Geometry: see drawing. Coordinates: mm, zero at the bounding-box minimum. A direction names the side the tool comes from. Coordinates: 2 decimals unless noted, no trailing zeros. Order: outer loops, then holes, each group sorted by start corner. A loop starts at its lowest first (then second) coordinate and runs counter-clockwise, first axis right, second up. Notation, with made-up numbers: (43.5, 49) -> (100.5, 49) arc R16 cw to (100.5, 70) -> close; hole circle Ø4 at (84, 40.5). An arc over 180 degrees is marked (long way). Use one line per item in the form item = value.
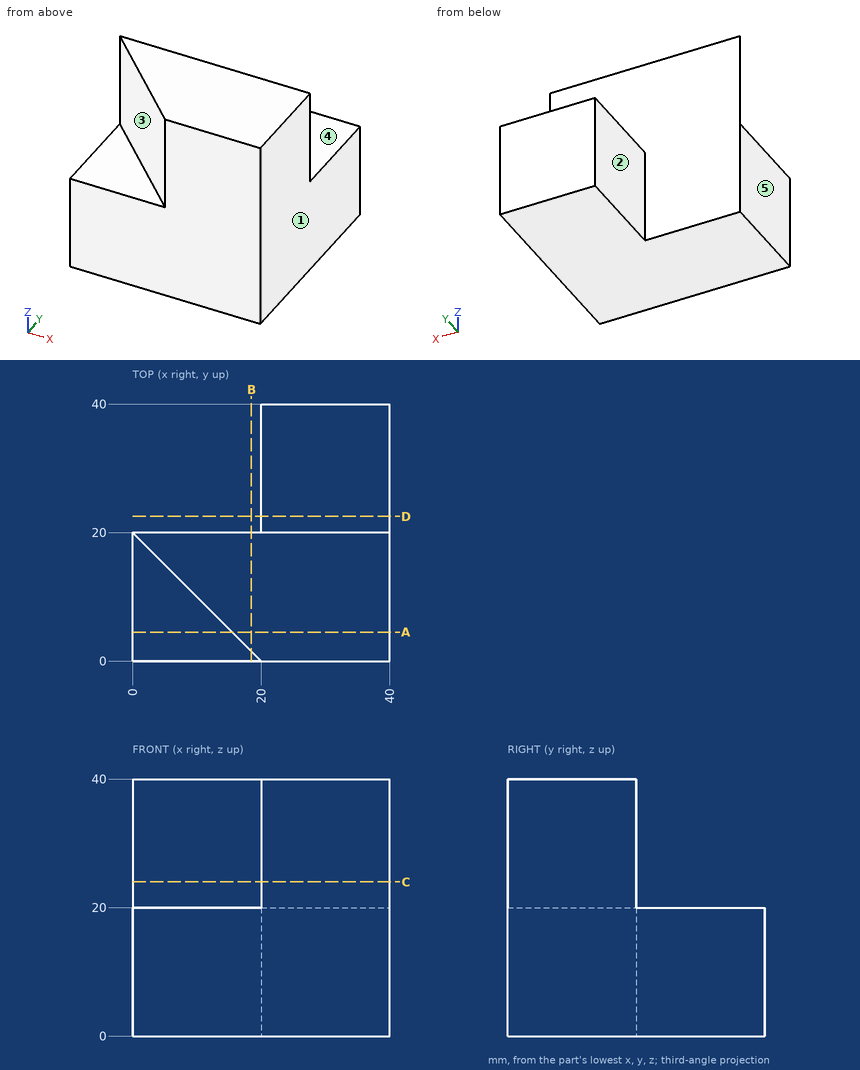
1) Contact query for flat-ended pins moving along their axis: P1, Ø16, axis at y = 31, z = 10.5, coming from the -X side; P2, Ø12, axis at x = 9.5, y = 6.5, coming from the -Z side; P3, Ø6, axis at x = 34, y = 25, coming from the +Z side; P4, Ø12, axis at y = 29.5, z = 30, coming from the -X side. Output: stop coordinate, or through.
Results found:
P1 = 20
P2 = 0
P3 = 20
P4 = through
2) Material intervals for probe 1 along Z at (x, y) = (11, 7.5); probe 2 along X at (y, z) = (27, 8.5), sorted ascending. Write a range as from..to.
Results found:
probe_1 = 0..20
probe_2 = 20..40
3) Section B-B, the plane x = 18.5. Output: boundary loops of the cut face in (y, z).
Results found:
outline = (0, 0) -> (20, 0) -> (20, 40) -> (1.5, 40) -> (1.5, 20) -> (0, 20) -> close
4) Access query for the marked faces 1, 2, 3, 4 and 5. Directions: +Z, -Z, +X, -X, +Y, -Y. A direction counts if a zero-diameter tool reaches every point of the face in a straight line with its end or side. Return the directions, or none.
Results found:
face_1 = +Z, -Z, +X, +Y, -Y
face_2 = +Z, -Z, -X, +Y
face_3 = +Z, -X, -Y
face_4 = +Z, +X, -X, +Y
face_5 = +Z, -Z, -X, +Y, -Y
5) Section C-C, the plane z = 24. Output: boundary loops of the cut face in (x, y).
Results found:
outline = (0, 20) -> (20, 0) -> (40, 0) -> (40, 20) -> close
6) Section D-D, the plane y = 22.5. Output: boundary loops of the cut face in (x, z).
Results found:
outline = (20, 0) -> (40, 0) -> (40, 20) -> (20, 20) -> close
7) Section A-A, the plane y = 4.5. Output: boundary loops of the cut face in (x, z).
Results found:
outline = (0, 0) -> (40, 0) -> (40, 40) -> (15.5, 40) -> (15.5, 20) -> (0, 20) -> close
